The listing builds one solid part. Answer for the finished solid, in the listing's coordinates (mm). A direction names the side the tool comes from. Give positions to 0.01 mm unless a question says otherwise; leave off trailing zeros. Loops run counter-clockwise (first coordinate to the right, second up) from the corner with the lowest first, then second, coordinate; pieces in that order, holes last. Notation, with made-up numbers: M 50,-6.75 L 61,-6.75 A31 ccw 61,24.25 Z; hole C 81,-4 d10. An arc over 180 degrees is marked long. Use one line per item in the form item = value. Start each with the question number.
1. The part is cut by section C-C (z = 2.75). Write down the section's boundary in (x, y), and give its area (3 significant figures).
2. Each of these flat-tipped pins is pushed along its axis until it touches: pin 1 Ø2 at (x, y) = (7.5, -2.5) entering from +Z; pin 2 Ø8 at (x, z) = (9, -0.5) entering from +Y; pin 3 Ø2 at (x, y) = (-8, -3.5) entering from -Z. Where does it stop, or does it pass through?
3. The part is cut by section D-D (y = -5.5). Write down the section's boundary in (x, z).
4. The part is cut by section B-B (x = 0). Write down the section's boundary in (y, z), and give its area (3 significant figures).
5. The part is cut by section A-A (z = -1.25). Write down the section's boundary in (x, y), and give its area (3 significant figures).
6. For faces 4 (the face through (0, 0, -5)), 5 (the face through (-7, -4, -2)), 6 (the face through (-7, -3, -5)), determine the directions among +Z, -Z, +X, -X, +Y, -Y from which every point of the face is accessible in a straight line to the end or side of a thin tool.
7. Straight lines are drawn through the part: line 1 (Z direction, x = -6.5, y = -2.25); line 2 (X direction, y = -3.5, z = -3.25); line 3 (Y direction, x = -3, z = -5.75). For each, find the intervals that lie inside material, in ascending order. Write a range as from..to.
8. The mould has two halves that part along Y. Classify faces 1 (the face through (-11.442, -3.103, -3.479)), 2 (the face through (-4.78, -3.42, -5.49)), 3 (the face through (-2.852, 2.805, -5.507)): released by +Y, released by -Y, zero draft, split by the parting line, or undercut.
from build123d import *

# Parameters (mm, degrees)
F0_W      = 12.5
F0_H      = 13.5
F0_R      = 5.75
F1_DEPTH  = 5
F3_DEPTH  = 5
F5_DEPTH  = 25
F6_R      = 1.5
F7_DEPTH  = 5
F9_DEPTH  = 1
F10_R     = 1.5
F11_DEPTH = 2
F13_W     = 6.183999799
F13_H     = 4
F14_DEPTH = 25
F17_DEPTH = 10
F20_DEPTH = 25
F21_R     = 3.5
F22_DEPTH = 3


# Not quite as in the source:
# - a feature of the source that left no trace in its solid (it failed there, or was rolled back) is left out
# - a feature names something its author has since deleted; it is built from what else it names


with BuildPart() as f1:
    # F0 (on Top) → F1 (new body, symmetric)
    with BuildSketch(Plane.XY):
        Rectangle(F0_W, F0_H)
        Circle(F0_R, mode=Mode.SUBTRACT)
    extrude(amount=F1_DEPTH, both=True)

    # F2 (on Top) → F3 (join, symmetric)
    with BuildSketch(Plane.XY):
        with BuildLine():
            Line((-4.7552825815, 3.4549150281), (-7.2654252801, 0))
            Line((-7.2654252801, 0), (-4.7552825815, -3.4549150281))
            ThreePointArc((-4.7552825815, -3.4549150281), (-5.8778525229, 0), (-4.7552825815, 3.4549150281))
        make_face()
        with BuildLine():
            Line((4.7552825815, -3.4549150281), (7.2654252801, 0))
            Line((7.2654252801, 0), (4.7552825815, 3.4549150281))
            ThreePointArc((4.7552825815, 3.4549150281), (5.8778525229, 0), (4.7552825815, -3.4549150281))
        make_face()
    extrude(amount=F3_DEPTH, both=True)

    # F4 (on face) → F5 (cut)
    with BuildSketch(Plane.XY.offset(5)):
        Polygon((-8.2530292036, 7.939198947), (-6.25, 1.3976129971), (-1.4972596068, 7.939198947), align=None)
        Polygon((-1.4972596068, -7.939198947), (-6.25, -1.3976129971), (-8.2530292036, -7.939198947), align=None)
        Polygon((8.2530292036, -7.939198947), (6.25, -1.3976129971), (1.4972596068, -7.939198947), align=None)
        Polygon((1.4972596068, 7.939198947), (6.25, 1.3976129971), (8.2530292036, 7.939198947), align=None)
    extrude(amount=-F5_DEPTH, mode=Mode.SUBTRACT)

    # F6 (on Top) → F7 (join, symmetric)
    with BuildSketch(Plane.XY):
        with BuildLine():
            Line((-7.2654252801, 0), (-10.173537518, -1.1373915846))
            ThreePointArc((-10.173537518, -1.1373915846), (-11.4402841733, -3.138029064), (-9.9101168699, -4.9451774907))
            Line((-9.9101168699, -4.9451774907), (-2.5670624157, -6.7007963666))
            Line((-2.5670624157, -6.7007963666), (-2.361263216, -6.75))
            Line((-2.361263216, -6.75), (-7.2654252801, 0))
        make_face()
        with Locations((-9.4450528641, -3)):
            Circle(F6_R, mode=Mode.SUBTRACT)
    extrude(amount=F7_DEPTH, both=True)

    # F8 (on face) → F9 (join)
    with BuildSketch(Plane(origin=(0, 0, -5), x_dir=(1, 0, 0), z_dir=(0, 0, -1))):
        Polygon((2.361263216, -6.75), (7.2654252801, 0), (2.361263216, 6.75), (-2.361263216, 6.75), (-7.2654252801, 0), (-2.361263216, -6.75), align=None)
    extrude(amount=F9_DEPTH)

    # F10 (on Top) → F11 (join, symmetric)
    with BuildSketch(Plane.XY):
        with BuildLine():
            Line((7.2654252801, 0), (2.361263216, -6.75))
            Line((2.361263216, -6.75), (9.9101168699, -4.9451774907))
            ThreePointArc((9.9101168699, -4.9451774907), (11.4402841733, -3.138029064), (10.173537518, -1.1373915846))
            Line((10.173537518, -1.1373915846), (7.2654252801, 0))
        make_face()
        with Locations((9.4450528641, -3)):
            Circle(F10_R, mode=Mode.SUBTRACT)
    extrude(amount=F11_DEPTH, both=True)

    # F13 (on face) → F14 (cut)
    with BuildSketch(Plane(origin=(2.3481090856, -2.7983674386, 0), x_dir=(-0.7660444431, -0.6427876097, 0), z_dir=(-0.6427876097, 0.7660444431, 0))):
        with Locations((9.2396488302, 0)):
            Rectangle(F13_W, F13_H)
    extrude(amount=F14_DEPTH, mode=Mode.SUBTRACT)

    # F16 (on face) → F17 (cut)
    with BuildSketch(Plane.XY.offset(5)):
        Polygon((-6.5190746712, 6.3958671101), (-8.2398039802, 3.9384109772), (-3.2558972089, 0.4486418862), (-1.5351678999, 2.906098019), align=None)
        Polygon((8.2398039802, 3.9384109772), (6.5190746712, 6.3958671101), (1.5351678999, 2.906098019), (3.2558972089, 0.4486418862), align=None)
    extrude(amount=-F17_DEPTH, mode=Mode.SUBTRACT)

    # F19 (on face) → F20 (cut)
    with BuildSketch(Plane(origin=(0, 0, -6), x_dir=(1, 0, 0), z_dir=(0, 0, -1))):
        with BuildLine():
            ThreePointArc((-3.4186985828, 0.75), (-2.4748737342, 2.4748737342), (-0.75, 3.4186985828))
            Line((-0.75, 3.4186985828), (-0.75, 3.9290584114))
            ThreePointArc((-0.75, 3.9290584114), (-2.8284271247, 2.8284271247), (-3.9290584114, 0.75))
            Line((-3.9290584114, 0.75), (-3.4186985828, 0.75))
        make_face()
        with BuildLine():
            Line((0.75, 3.9290584114), (0.75, 3.4186985828))
            ThreePointArc((0.75, 3.4186985828), (2.4748737342, 2.4748737342), (3.4186985828, 0.75))
            Line((3.4186985828, 0.75), (3.9290584114, 0.75))
            ThreePointArc((3.9290584114, 0.75), (2.8284271247, 2.8284271247), (0.75, 3.9290584114))
        make_face()
        with BuildLine():
            Line((-0.75, -3.9290584114), (-0.75, -3.4186985828))
            ThreePointArc((-0.75, -3.4186985828), (-2.4748737342, -2.4748737342), (-3.4186985828, -0.75))
            Line((-3.4186985828, -0.75), (-3.9290584114, -0.75))
            ThreePointArc((-3.9290584114, -0.75), (-2.8284271247, -2.8284271247), (-0.75, -3.9290584114))
        make_face()
        with BuildLine():
            ThreePointArc((3.4186985828, -0.75), (2.4748737342, -2.4748737342), (0.75, -3.4186985828))
            Line((0.75, -3.4186985828), (0.75, -3.9290584114))
            ThreePointArc((0.75, -3.9290584114), (2.8284271247, -2.8284271247), (3.9290584114, -0.75))
            Line((3.9290584114, -0.75), (3.4186985828, -0.75))
        make_face()
    extrude(amount=-F20_DEPTH, mode=Mode.SUBTRACT)

    # F21 (on face) → F22 (join)
    with BuildSketch(Plane(origin=(0, 0, -6), x_dir=(1, 0, 0), z_dir=(0, 0, -1))):
        Circle(F21_R)
    extrude(amount=F22_DEPTH)


solid = f1.part
Derived:
q1.outline = M -10.17,-1.14 A2 ccw -9.91,-4.95 L -2.36,-6.75 L 2.36,-6.75 L 7.27,0 L 5.7,2.16 L 5.41,1.96 A5.75 cw long -5.41,1.96 L -5.7,2.16 L -7.27,0 Z; M -3.93,4.59 L -3.69,4.41 A5.75 cw 3.69,4.41 L 3.93,4.59 L 2.36,6.75 L -2.36,6.75 Z; hole C -9.45,-3 d3
q1.area = 48.5 mm2
q2.pin_1 = 2
q2.pin_2 = 2.16
q2.pin_3 = -5
q3.outline = M -7.59,-5 L -3.27,-5 L -3.27,-6 L 3.27,-6 L 3.27,-2 L 7.59,-2 L 7.59,2 L 3.27,2 L 3.27,5 L 1.68,5 L 1.68,-5 L -1.68,-5 L -1.68,5 L -7.59,5 L -7.59,2 L -3.41,2 L -3.41,-2 L -7.59,-2 Z
q4.outline = M -6.75,-6 L -3.5,-6 L -3.5,-9 L 3.5,-9 L 3.5,-6 L 6.75,-6 L 6.75,5 L 5.75,5 L 5.75,-5 L -5.75,-5 L -5.75,5 L -6.75,5 Z
q4.area = 54.5 mm2
q5.outline = M -7.84,-0.22 L -2.36,-6.75 L 2.36,-6.75 L 9.91,-4.95 A2 ccw 10.17,-1.14 L 7.27,0 L 5.7,2.16 L 5.41,1.96 A5.75 cw long -5.41,1.96 L -5.7,2.16 L -7.27,0 Z; M -3.93,4.59 L -3.69,4.41 A5.75 cw 3.69,4.41 L 3.93,4.59 L 2.36,6.75 L -2.36,6.75 Z; hole C 9.45,-3 d3
q5.area = 51.0 mm2
q6.face_4 = +Z
q6.face_5 = -X, -Y
q6.face_6 = -Z, -X, -Y
q7.line_1 = -5..-2, 2..5
q7.line_2 = -11.38..-10.86, -8.03..-4.56, 4.56..4.72
q7.line_3 = -5.87..-2.65, -1.8..1.8, 2.65..5.87
q8.face_1 = split by the parting line
q8.face_2 = released by -Y
q8.face_3 = undercut
